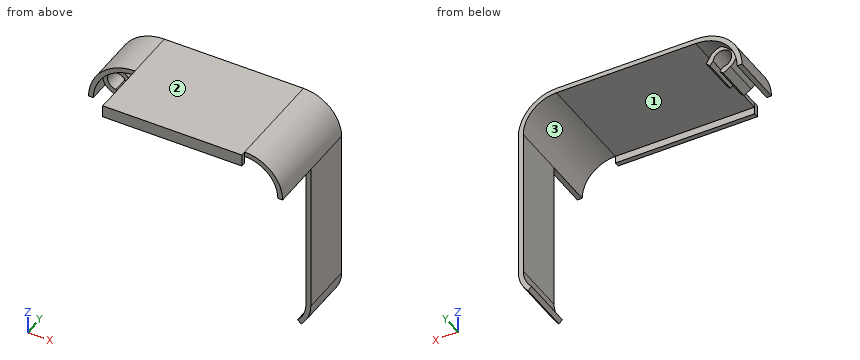
from build123d import *

# Parameters (mm, degrees)
EXTRUDE_THIN1_DEPTH = 53.975
BOSS_EXTRUDE1_START = 30.48
BOSS_EXTRUDE1_DEPTH = 19.05
SKETCH12_W          = 34.867415814
SKETCH12_H          = 30.456007234
CUT_EXTRUDE1_DEPTH  = 27.000736901
BOSS_EXTRUDE2_DEPTH = 28.194
SKETCH15_W          = 72.898
SKETCH15_H          = 6.35
BOSS_EXTRUDE3_DEPTH = 2.54


with BuildPart() as part:
    # Sketch8 → Extrude-Thin1 (new body)
    with BuildSketch(Plane(origin=(0, 0, 0), x_dir=(1, 0, 0), z_dir=(0, 1, 0))):
        with BuildLine():
            ThreePointArc((-21.840673053, -0.381230366), (-15.310661969, -15.580242811), (0, -21.844))
            Line((0, -21.844), (72.898, -21.844))
            ThreePointArc((72.898, -21.844), (85.209931142, -16.744231142), (90.3097, -4.4323))
            Line((90.3097, -4.4323), (92.8497, -4.4323))
            ThreePointArc((92.8497, -4.4323), (87.005982366, -18.540282366), (72.898, -24.384))
            Line((72.898, -24.384), (0, -24.384))
            ThreePointArc((0, -24.384), (-17.090971501, -17.391898952), (-24.380286199, -0.425559479))
            Line((-24.380286199, -0.425559479), (-21.840673053, -0.381230366))
        make_face()
    extrude(amount=EXTRUDE_THIN1_DEPTH)

    # Sketch10 → Boss-Extrude1 (add)
    with BuildSketch(Plane(origin=(0, 0, 0), x_dir=(1, 0, 0), z_dir=(0, 1, 0)).offset(BOSS_EXTRUDE1_START)):
        with BuildLine():
            Line((-6.641231784, -11.936352934), (-4.843541474, -10.138662625))
            Line((-4.843541474, -10.138662625), (-3.045851165, -11.936352934))
            Line((-3.045851165, -11.936352934), (-5.383859486, -15.696211745))
            ThreePointArc((-5.383859486, -15.696211745), (-7.807213542, -17.931410627), (-10.959862847, -18.895548216))
            ThreePointArc((-10.959862847, -18.895548216), (-15.446040528, -15.446040528), (-18.895548216, -10.959862847))
            ThreePointArc((-18.895548216, -10.959862847), (-17.931410627, -7.807213542), (-15.696211745, -5.383859486))
            Line((-15.696211745, -5.383859486), (-11.936352934, -3.045851165))
            Line((-11.936352934, -3.045851165), (-10.138662625, -4.843541474))
            Line((-10.138662625, -4.843541474), (-11.936352934, -6.641231784))
            ThreePointArc((-11.936352934, -6.641231784), (-14.946738288, -14.946738288), (-6.641231784, -11.936352934))
        make_face()
    extrude(amount=BOSS_EXTRUDE1_DEPTH)

    # Sketch12 → Cut-Extrude1 (cut, through all)
    with BuildSketch(Plane(origin=(0, 0, 0), x_dir=(-0.999847695, 0, 0.017452406), z_dir=(-0.017452406, 0, -0.999847695))):
        with Locations((17.814938273, 11.759496383)):
            Rectangle(SKETCH12_W, SKETCH12_H)
    extrude(amount=-CUT_EXTRUDE1_DEPTH, mode=Mode.SUBTRACT)

    # Sketch14 → Boss-Extrude2 (add)
    with BuildSketch(Plane(origin=(0, 53.975, 0), x_dir=(1, 0, 0), z_dir=(0, 1, 0))):
        with BuildLine():
            Line((85.945696481, 85.211636481), (87.741747705, 87.007687705))
            ThreePointArc((87.741747705, 87.007687705), (91.52218645, 81.349861294), (92.8497, 74.676))
            Line((92.8497, 74.676), (92.8497, -4.4323))
            Line((92.8497, -4.4323), (90.3097, -4.4323))
            Line((90.3097, -4.4323), (90.3097, 74.676))
            ThreePointArc((90.3097, 74.676), (89.175532438, 80.377845376), (85.945696481, 85.211636481))
        make_face()
    extrude(amount=-BOSS_EXTRUDE2_DEPTH)

    # Sketch15 → Boss-Extrude3 (add)
    with BuildSketch(Plane.XZ):
        with Locations((36.449, 21.209)):
            Rectangle(SKETCH15_W, SKETCH15_H)
    extrude(amount=BOSS_EXTRUDE3_DEPTH)


solid = part.part
Source: CAD feature listing. Evaluate the final solid. Frame: model axes, mm. Face numbers are marked on the shaded views. Round coordinates to 2 decimals unless told otherwise and drop trailing zeros. Write each loop counter-clockwise with the first axis right and the second up, starting at its lowest first coordinate (ties: lowest second). Pieces come first, ordered by that corner, then holes. Notation, with made-up numbers: M -8.5,17 L 28.5,17 A34 ccw 28.5,49 Z; hole C -16.5,54 d3. An arc over 180 degrees is marked long. One line per item, written item: value. Start each with the question number.
Item 1: Section query B-B (x = 43.5). Return the cut outline in (y, z) (3 decimals).
Item 2: Section query D-D (y = 6.5). Return the cut outline in (x, z).
Item 3: Ray query, L1, parallel to Z at x = 62.5, y = 20; L2, parallel to X at y = 43.5, z = -46.5; L3, parallel to Z at x = -11.5, y = 48.5. Return the intervals inside material, ascending. Write a range as from..to.
Item 4: Mould query, pull axis Z, two halves, no side actions, for the marked faces 1, 2 and 3. Classes: pulls with the +Z half, pulls with the -Z half, needs draft (parallel to the pull), parting line crosses it, or undercut.
Item 5: Pin query (flat end, axial travel): pin 1 (1.5 mm diameter, centred on x = 5, y = 12, fed in from -Z); pin 2 (14 mm diameter, centred on y = 36, z = -23, fed in from -X); pin 3 (5 mm diameter, centred on x = -10.5, z = 14.5, fed in from +Y); pin 4 (15.5 mm diameter, centred on x = -11.5, z = 11.5, fed in from +Y) (3 decimals). Return the tip coordinate at first contact, or that it passes through.
Item 6: Section query A-A (y = 37). Return the cut outline in (x, z).
Item 7: Section query C-C (z = -38.5). Return the cut outline in (x, y) (3 decimals), plus the area to 3 significant figures.
Result set:
1. outline: M -2.54,18.034 L 0,18.034 L 0,21.844 L 53.975,21.844 L 53.975,24.384 L -2.54,24.384 Z
2. outline: M 0,21.84 L 72.9,21.84 A17.41 cw 90.31,4.43 L 92.85,4.43 A19.95 ccw 72.9,24.38 L 0.04,24.38 Z
3. L1: z = 21.84..24.38
3. L2: x = 90.31..92.85
3. L3: z = 3.48..6.2, 16.38..21.5
4. face 1: pulls with the -Z half
4. face 2: pulls with the +Z half
4. face 3: undercut
5. pin 1: stops at z = 21.84
5. pin 2: stops at x = 90.31
5. pin 3: stops at y = 49.53
5. pin 4: stops at y = 53.975
6. outline: M -24.38,0.43 L -21.84,0.38 A21.84 cw -18.9,10.96 A7.42 ccw -15.7,5.38 L -11.94,3.05 L -10.14,4.84 L -11.94,6.64 A4.88 cw long -6.64,11.94 L -4.84,10.14 L -3.05,11.94 L -5.38,15.7 A7.42 ccw -10.96,18.9 A21.84 cw 0,21.84 L 72.9,21.84 A17.41 cw 90.31,4.43 L 90.31,-74.68 A14.9 cw 85.95,-85.21 L 87.74,-87.01 A17.44 ccw 92.85,-74.68 L 92.85,4.43 A19.95 ccw 72.9,24.38 L 0,24.38 A24.38 ccw Z
7. outline: M 90.31,25.781 L 92.85,25.781 L 92.85,53.975 L 90.31,53.975 Z
7. area: 71.6 mm²
